Geometry: final body of the model. Coordinates: model frame, mm. A direction names the side the tool comes from. Coordinates: 2 decimals unless noted, no trailing zeros. Write each loop counter-clockwise with the first axis right and the second up, starting at its lowest first coordinate (ties: lowest second). Pieces come first, ordered by that corner, then holes.
from build123d import *

# Parameters (mm, degrees)
SKETCH1_W           = 43
SKETCH1_H           = 40
BOSS_EXTRUDE1_DEPTH = 15
SKETCH3_W           = 5.1
SKETCH3_H           = 6.605333129
CUT_EXTRUDE1_DEPTH  = 3
SKETCH3_4_W         = 5.2
SKETCH3_4_H         = 16.040940276
CUT_EXTRUDE2_DEPTH  = 10


with BuildPart() as part:
    # Sketch1 → Boss-Extrude1 (new body)
    with BuildSketch(Plane.XY):
        with Locations((1.748803828, 1.277511962)):
            Rectangle(SKETCH1_W, SKETCH1_H)
    extrude(amount=BOSS_EXTRUDE1_DEPTH)

    # Sketch3 → Cut-Extrude1 (cut)
    with BuildSketch(Plane.XY.offset(15)):
        with Locations((-0.801196172, 17.974845398)):
            Rectangle(SKETCH3_W, SKETCH3_H)
        with Locations((4.298803828, 17.974845398)):
            Rectangle(SKETCH3_W, SKETCH3_H)
    extrude(amount=-CUT_EXTRUDE1_DEPTH, mode=Mode.SUBTRACT)

    # Sketch3_4 → Cut-Extrude2 (cut)
    with BuildSketch(Plane.XY.offset(15)):
        with Locations((-12.051196172, -10.7020179)):
            Rectangle(SKETCH3_4_W, SKETCH3_4_H)
        with Locations((15.548803828, -10.7020179)):
            Rectangle(SKETCH3_4_W, SKETCH3_4_H)
    extrude(amount=-CUT_EXTRUDE2_DEPTH, mode=Mode.SUBTRACT)


solid = part.part
Item 1: Section B-B, the plane z = 13.5. Output: boundary loops of the cut face in (x, y), plus the area to 3 significant figures.
Derived:
outline: (-19.75, -18.72) - (-14.65, -18.72) - (-14.65, -2.68) - (-9.45, -2.68) - (-9.45, -18.72) - (12.95, -18.72) - (12.95, -2.68) - (18.15, -2.68) - (18.15, -18.72) - (23.25, -18.72) - (23.25, 21.28) - (6.85, 21.28) - (6.85, 14.67) - (-3.35, 14.67) - (-3.35, 21.28) - (-19.75, 21.28) - close
area: 1,490 mm2
Item 2: Material intervals for probe 1 along X at (y, z) = (-15.5, 10.75); probe 2 along X at (y, z) = (16, 13.5); probe 3 along Z at (x, y) = (15.5, -7), sorted ascending.
Derived:
probe 1: x = -19.75 to -14.65, -9.45 to 12.95, 18.15 to 23.25
probe 2: x = -19.75 to -3.35, 6.85 to 23.25
probe 3: z = 0 to 5
Item 3: Pull-direction query (X, two-part tool) for faces 4 (the flat face through (-19.751, 1, 7)), 5 (the flat face through (-12, -11, 5)), 6 (the flat face through (1, 2, 15)); classes: released by +X, released by -X, zero draft, split by the parting line, or undercut.
Derived:
face 4: released by -X
face 5: undercut
face 6: zero draft
Item 4: Section D-D, the plane z = 6.5. Output: boundary loops of the cut face in (x, y), plus the area to 3 significant figures.
Derived:
outline: (-19.75, -18.72) - (-14.65, -18.72) - (-14.65, -2.68) - (-9.45, -2.68) - (-9.45, -18.72) - (12.95, -18.72) - (12.95, -2.68) - (18.15, -2.68) - (18.15, -18.72) - (23.25, -18.72) - (23.25, 21.28) - (-19.75, 21.28) - close
area: 1,550 mm2
Item 5: Section A-A, the plane y = -9. Output: boundary loops of the cut face in (x, z).
Derived:
outline: (-19.75, 0) - (23.25, 0) - (23.25, 15) - (18.15, 15) - (18.15, 5) - (12.95, 5) - (12.95, 15) - (-9.45, 15) - (-9.45, 5) - (-14.65, 5) - (-14.65, 15) - (-19.75, 15) - close
Item 6: Pin query (flat end, axial travel): pin 1 (2.5 mm diameter, centred on x = 14.5, z = 9.5, fed in from -Y); pin 2 (1.6 mm diameter, centred on x = -12.5, y = -9, fed in from +Z); pin 3 (3.5 mm diameter, centred on x = 0, z = 14, fed in from +Y). Return the tip coordinate at first contact, or that it passes through.
Derived:
pin 1: stops at y = -2.68
pin 2: stops at z = 5
pin 3: stops at y = 14.67
Item 7: Section C-C, the plane x = 2.5. Output: boundary loops of the cut face in (y, z), plus the area to 3 significant figures.
Derived:
outline: (-18.72, 0) - (21.28, 0) - (21.28, 12) - (14.67, 12) - (14.67, 15) - (-18.72, 15) - close
area: 580 mm2
Item 8: Set-up query: faces 1 (the flat face through (1, -18.722, 7)), 2 (the flat face through (2, 18, 12)), 3 (the flat face through (-12, -2.682, 10)). Return all of +Z, -Z, +X, -X, +Y, -Y with unobstructed straight access to the full face (end or side cutting, diameter ignored); none if empty.
Derived:
face 1: +Z, -Z, +X, -X, -Y
face 2: +Z, +Y
face 3: +Z, -Y
